Check sheet for the modelled part. Datum: model origin and axes. Units: mm. A direction names the side the tool comes from. Round coordinates to 2 decimals unless told otherwise and drop trailing zeros. Order: outer loops, then holes, each group sorted by start corner. A loop starts at its lowest first (then second) coordinate and runs counter-clockwise, first axis right, second up. Notation, with made-up numbers: (64.5, 44.5) -> (75.5, 44.5) arc R24 ccw to (75.5, 73.5) -> close; hole circle Ø3 at (-14.5, -15.5). An arc over 180 degrees is marked (long way). Answer in a Markdown table with one row per item. Add a question column.
1. Sectioned sample at A-A, the plane x = 3.2. Record the boundary of the cut face in (y, z).
2. Sectioned sample at C-C, the plane y = 0.85. Record the boundary of the cut face in (x, z).
3. Draft check along X on faces 4 (the cylindrical face through (4.19, 0.04, 1.17)), 5 (the flat face through (0, 0, 2.15)), 6 (the flat face through (-3, 0, 2.6)), 7 (the flat face through (6.35, 0, 1)). Enter one of: +X half, -X half, draft (parallel to the pull), parting line (faces both ways), or undercut.
4. Access from +Z, -Z, +X, -X, +Y, -Y to the whole of each face (thin tool, end or side, straight path). Record for faces 1 (the flat face through (0, 0, 0)), 2 (the flat face through (5, 0, 2.15)), 3 (the flat face through (-5, 0, 2.15)).
5. Sectioned sample at B-B, the plane z = 1.3. Record the boundary of the cut face in (x, y), then the cut area to 3 significant figures.
6. Sectioned sample at D-D, the plane x = -0.5. Record the boundary of the cut face in (y, z).
7. Material ranges on L1, parallel to X at y = -0.15, z = 1.3; L2, parallel to X at y = 0.25, z = 0.7; L3, parallel to Y at x = 1.25, z = 0.5, recorded low to high. Write a range as from..to.
8. Depth check by flat-ended pin: P1, Ø1.5, axis at x = 0.5, y = 1.5, coming from the +Z side; P2, Ø1.4, axis at x = -0.5, z = 1, coming from the -Y side; P3, Ø0.5, axis at x = 0, z = 1, coming from the +Y side. Enter the tip coordinate at first touch or a pass-through.
```python
from build123d import *

# Parameters (mm, degrees)
SALIENTE_EXTRUIR1_DEPTH = 2.6
CROQUIS2_R              = 1
CORTAR_EXTRUIR1_DEPTH   = 3
CROQUIS4_W              = 3.7
CROQUIS4_H              = 0.1
SALIENTE_EXTRUIR2_DEPTH = 0.8
CHAFL_N1_SIZE           = 0.15
CROQUIS5_W              = 3.8
CROQUIS5_H              = 5.8
CROQUIS5_W_2            = 1.75
CORTAR_EXTRUIR2_DEPTH   = 0.45


with BuildPart() as part:
    # Croquis1 → Saliente-Extruir1 (new body)
    with BuildSketch(Plane.XY):
        Polygon((-1.85, 2.8), (1.85, 2.8), (1.85, 2.9), (6.35, 2.9), (6.35, -2.9), (1.85, -2.9), (1.85, -2.8), (-1.85, -2.8), (-1.85, -2.9), (-6.35, -2.9), (-6.35, 2.9), (-1.85, 2.9), align=None)
    extrude(amount=SALIENTE_EXTRUIR1_DEPTH)

    # Croquis2 → Cortar-Extruir1 (cut, symmetric)
    with BuildSketch(Plane(origin=(0, 0, 0), x_dir=(1, 0, 0), z_dir=(0, 1, 0))):
        with Locations(Location((-3.2, -1.3, 0), (0, 0, 270))):
            Circle(CROQUIS2_R)
        with Locations(Location((3.2, -1.3, 0), (0, 0, 270))):
            Circle(CROQUIS2_R)
    extrude(amount=CORTAR_EXTRUIR1_DEPTH, both=True, mode=Mode.SUBTRACT)

    # Croquis4 → Saliente-Extruir2 (add)
    with BuildSketch(Plane.XY.offset(2.6)):
        with Locations((0, 2.85)):
            Rectangle(CROQUIS4_W, CROQUIS4_H)
        with Locations((0, -2.85)):
            Rectangle(CROQUIS4_W, CROQUIS4_H)
    extrude(amount=-SALIENTE_EXTRUIR2_DEPTH)

    # Chaflán1
    # the kernel refuses this chamfer: 0.15 mm, written as the material it takes off along each edge
    with BuildSketch(Plane(origin=(-1.85, -2.9, 1.8), x_dir=(0, -0.027495876610587378, 0.9996219169112965), z_dir=(1, 0, 0))) as chafl_n1_piece_1_section:
        Polygon((CHAFL_N1_SIZE * 0.999621916911, -CHAFL_N1_SIZE * 0.0274958766106), (-CHAFL_N1_SIZE * 0.0274958766106, -CHAFL_N1_SIZE * 0.999621916911), (0, 0), align=None)
    chafl_n1_piece_1 = extrude(amount=3.7, mode=Mode.PRIVATE)
    chafl_n1_piece_1 = split(chafl_n1_piece_1, bisect_by=Plane(origin=(0, -2.8, 1.85460455), z_dir=(0, -1, 0)), keep=Keep.TOP, mode=Mode.PRIVATE)
    add(chafl_n1_piece_1, mode=Mode.SUBTRACT)
    with BuildSketch(Plane(origin=(1.85, 2.9, 1.8), x_dir=(0, 0.027495876610587378, 0.9996219169112965), z_dir=(-1, 0, 0))) as chafl_n1_piece_2_section:
        Polygon((CHAFL_N1_SIZE * 0.999621916911, -CHAFL_N1_SIZE * 0.0274958766106), (-CHAFL_N1_SIZE * 0.0274958766106, -CHAFL_N1_SIZE * 0.999621916911), (0, 0), align=None)
    chafl_n1_piece_2 = extrude(amount=3.7, mode=Mode.PRIVATE)
    chafl_n1_piece_2 = split(chafl_n1_piece_2, bisect_by=Plane(origin=(0, 2.8, 1.85460455), z_dir=(0, 1, 0)), keep=Keep.TOP, mode=Mode.PRIVATE)
    add(chafl_n1_piece_2, mode=Mode.SUBTRACT)

    # Croquis5 → Cortar-Extruir2 (cut)
    with BuildSketch(Plane.XY.offset(2.6)):
        Rectangle(CROQUIS5_W, CROQUIS5_H)
        with Locations((-5.475, 0)):
            Rectangle(CROQUIS5_W_2, CROQUIS5_H)
        with Locations((5.475, 0)):
            Rectangle(CROQUIS5_W_2, CROQUIS5_H)
    extrude(amount=-CORTAR_EXTRUIR2_DEPTH, mode=Mode.SUBTRACT)


solid = part.part
```
Answer key:
| question | item | result |
|---|---|---|
| 1 | outline | (-2.9, 0) -> (2.9, 0) -> (2.9, 0.3) -> (-2.9, 0.3) -> close; (-2.9, 2.3) -> (2.9, 2.3) -> (2.9, 2.6) -> (-2.9, 2.6) -> close |
| 2 | outline | (-6.35, 0) -> (6.35, 0) -> (6.35, 2.15) -> (4.6, 2.15) -> (4.6, 2.6) -> (1.9, 2.6) -> (1.9, 2.15) -> (-1.9, 2.15) -> (-1.9, 2.6) -> (-4.6, 2.6) -> (-4.6, 2.15) -> (-6.35, 2.15) -> close; hole circle Ø2 at (-3.2, 1.3); hole circle Ø2 at (3.2, 1.3) |
| 3 | face 4 | undercut |
| 3 | face 5 | undercut |
| 3 | face 6 | draft |
| 3 | face 7 | +X half |
| 4 | face 1 | -Z, +X, -X, +Y, -Y |
| 4 | face 2 | +Z, +X, +Y, -Y |
| 4 | face 3 | +Z, -X, +Y, -Y |
| 5 | outline | (-6.35, -2.9) -> (-4.2, -2.9) -> (-4.2, 2.9) -> (-6.35, 2.9) -> close; (-2.2, -2.9) -> (-1.85, -2.9) -> (-1.85, -2.8) -> (1.85, -2.8) -> (1.85, -2.9) -> (2.2, -2.9) -> (2.2, 2.9) -> (1.85, 2.9) -> (1.85, 2.8) -> (-1.85, 2.8) -> (-1.85, 2.9) -> (-2.2, 2.9) -> close; (4.2, -2.9) -> (6.35, -2.9) -> (6.35, 2.9) -> (4.2, 2.9) -> close |
| 5 | area | 49.7 mm² |
| 6 | outline | (-2.9, 1.95) -> (-2.8, 1.85) -> (-2.8, 0) -> (2.8, 0) -> (2.8, 1.85) -> (2.9, 1.95) -> (2.9, 2.15) -> (-2.9, 2.15) -> close |
| 7 | L1 | x = -6.35..-4.2, -2.2..2.2, 4.2..6.35 |
| 7 | L2 | x = -6.35..-4, -2.4..2.4, 4..6.35 |
| 7 | L3 | y = -2.8..2.8 |
| 8 | P1 | stops at z = 2.15 |
| 8 | P2 | stops at y = -2.8 |
| 8 | P3 | stops at y = 2.8 |
